Geometry check sheet. Reference: the model listing, model coordinates, mm. Face numbers are marked on the shaded views. A direction names the side the tool comes from. Round coordinates to 2 decimals unless told otherwise and drop trailing zeros. Loops run counter-clockwise (first coordinate to the right, second up) from the corner with the lowest first, then second, coordinate; pieces in that order, holes last. Notation, with made-up numbers: (13, 21) - (42, 21) arc R27 cw to (42, 57) - close; hole circle Ø3 at (-38.5, 81.5). An arc over 180 degrees is marked (long way). Answer as CSV lines item,"result". Start each with the question number.
1) Thickness scan on line 1 along Y through (x, z) = (-40, 2); line 2 along X through (y, z) = (-0.5, 26); line 3 along Z through (x, y) = (2.5, -3.5). Record the ranges inside material, lowest first.
2) Cross-section at A-A on x = -8.5. Record the boundary of the cut face in (y, z).
3) Access from +Z, -Z, +X, -X, +Y, -Y to the whole of each face (thin tool, end or side, straight path). Record for the marked faces 1, 2 and 3.
4) Cross-section at B-B on y = -21. Record the boundary of the cut face in (x, z).
5) Cross-section at D-D on y = -14.5. Record the boundary of the cut face in (x, z).
6) Depth check by flat-ended pin: P1, Ø12, axis at y = -1, z = 16.5, coming from the +X side; P2, Ø5.5, axis at y = -2, z = 14, coming from the -X side; P3, Ø6.5, axis at x = 40, y = 21, coming from the +Z side. Enter the tip coordinate at first touch or a pass-through.
7) Draft check along X on the marked faces 4, 5, 6 and 7. Enter one of: released by +X, released by -X, zero draft, split by the parting line, or undercut.
8) Cross-section at C-C on z = 8.5. Record the boundary of the cut face in (x, y), and give its area (3 significant figures).
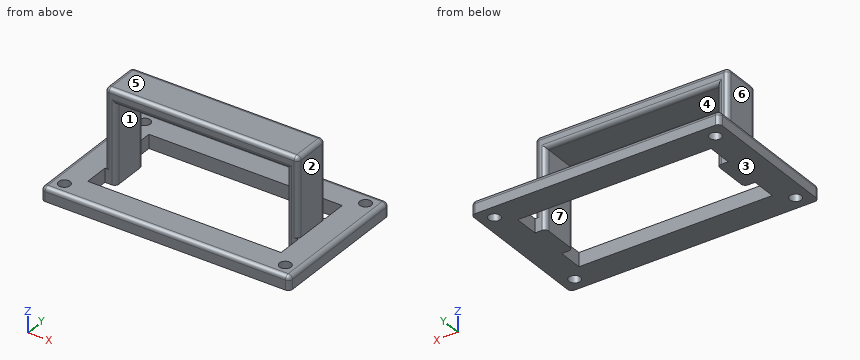
from build123d import *

# Parameters (mm, degrees)
SKETCH2_W                 = 52
SKETCH2_H                 = 90
BOSS_EXTRUDE1_DEPTH       = 5
BOSS_EXTRUDE2_DEPTH       = 14
M5X0_8_TAPPED_HOLE1_D     = 4.2
M5X0_8_TAPPED_HOLE1_DEPTH = 7.5
M5X0_8_TAPPED_HOLE1_TIP   = 1.2618073
FILLET1_R                 = 1.5


with BuildPart() as part:
    # Sketch2 → Boss-Extrude1 (new body)
    with BuildSketch(Plane(origin=(0, 0, 0), x_dir=(0, 1, 0), z_dir=(0, 0, 1))):
        Rectangle(SKETCH2_W, SKETCH2_H)
        Polygon((-16, 35), (-7, 35), (-7, 31), (7, 31), (7, 35), (16, 35), (16, -35), (7, -35), (7, -31), (-7, -31), (-7, -35), (-16, -35), align=None, mode=Mode.SUBTRACT)
    extrude(amount=BOSS_EXTRUDE1_DEPTH)

    # Sketch4 → Boss-Extrude2 (add)
    with BuildSketch(Plane.XZ.offset(7)):
        Polygon((-35, 5), (-35, 33.5), (35, 33.5), (35, 5), (31, 5), (31, 28.5), (-31, 28.5), (-31, 5), align=None)
    extrude(amount=-BOSS_EXTRUDE2_DEPTH)

    # M5x0.8 Tapped Hole1
    with Locations(Plane.XY.offset(5)):
        with Locations((-40, 21), (40, 21), (-40, -21), (40, -21)):
            Hole(M5X0_8_TAPPED_HOLE1_D / 2, depth=M5X0_8_TAPPED_HOLE1_DEPTH)
            with Locations((0, 0, -(M5X0_8_TAPPED_HOLE1_DEPTH + M5X0_8_TAPPED_HOLE1_TIP / 2))):  # 118° drill point
                Cone(0, M5X0_8_TAPPED_HOLE1_D / 2, M5X0_8_TAPPED_HOLE1_TIP, mode=Mode.SUBTRACT)

    # Fillet1
    fillet1_edges = [part.edges().sort_by_distance(p)[0] for p in [
        (0, 26, 5),
        (-45, 0, 5),
        (31, -7, 14.25),
        (31, 7, 14.25),
        (-31, 7, 14.25),
        (-31, -7, 14.25),
        (0, -26, 5),
        (-35, 7, 19.25),
        (0, 7, 33.5),
        (-35, 0, 33.5),
        (35, 7, 19.25),
        (35, 0, 33.5),
        (0, 7, 28.5),
        (0, -7, 28.5),
        (35, -7, 19.25),
        (0, -7, 33.5),
        (-35, -7, 19.25),
        (-45, -26, 2.5),
        (-45, 26, 2.5),
        (45, 26, 2.5),
        (45, -26, 2.5),
        (45, 0, 5),
    ]]
    fillet(fillet1_edges, radius=FILLET1_R)


solid = part.part
Answer block:
1,line 1,"y = -26 to -23.1, -18.9 to 18.9, 23.1 to 26"
1,line 2,"x = -35 to -31, 31 to 35"
1,line 3,"z = 28.5 to 33.5"
2,outline,"(-26, 0) - (-16, 0) - (-16, 5) - (-24.5, 5) arc R1.5 ccw to (-26, 3.5) - close; (-7, 30) arc R1.5 ccw to (-5.5, 28.5) - (5.5, 28.5) arc R1.5 ccw to (7, 30) - (7, 32) arc R1.5 ccw to (5.5, 33.5) - (-5.5, 33.5) arc R1.5 ccw to (-7, 32) - close; (16, 0) - (26, 0) - (26, 3.5) arc R1.5 ccw to (24.5, 5) - (16, 5) - close"
3,face 1,"-Z"
3,face 2,"+Z, +X, +Y, -Y"
3,face 3,"-Z, +X, -X, +Y, -Y"
4,outline,"(-45, 0) - (-42.1, 0) - (-42.1, 5) - (-43.5, 5) arc R1.5 ccw to (-45, 3.5) - close; (-37.9, 0) - (37.9, 0) - (37.9, 5) - (-37.9, 5) - close; (42.1, 0) - (45, 0) - (45, 3.5) arc R1.5 ccw to (43.5, 5) - (42.1, 5) - close"
5,outline,"(-45, 0) - (-35, 0) - (-35, 5) - (-43.5, 5) arc R1.5 ccw to (-45, 3.5) - close; (35, 0) - (45, 0) - (45, 3.5) arc R1.5 ccw to (43.5, 5) - (35, 5) - close"
6,P1,"stops at x = 35"
6,P2,"stops at x = -35"
6,P3,"stops at z = 5"
7,face 4,"undercut"
7,face 5,"zero draft"
7,face 6,"released by -X"
7,face 7,"undercut"
8,outline,"(-35, -5.5) arc R1.5 ccw to (-33.5, -7) - (-32.5, -7) arc R1.5 ccw to (-31, -5.5) - (-31, 5.5) arc R1.5 ccw to (-32.5, 7) - (-33.5, 7) arc R1.5 ccw to (-35, 5.5) - close; (31, -5.5) arc R1.5 ccw to (32.5, -7) - (33.5, -7) arc R1.5 ccw to (35, -5.5) - (35, 5.5) arc R1.5 ccw to (33.5, 7) - (32.5, 7) arc R1.5 ccw to (31, 5.5) - close"
8,area,"108 mm^2"
